Geometry check sheet. Reference: the model listing, model coordinates, mm. A direction names the side the tool comes from. Coordinates: 2 decimals unless noted, no trailing zeros. Loops run counter-clockwise (first coordinate to the right, second up) from the corner with the lowest first, then second, coordinate; pieces in that order, holes last. Notation, with made-up numbers: (60, 59) -> (99, 59) arc R25 ccw to (99, 79) -> close; hole circle Ø9 at (48.5, 49.5). An arc over 180 degrees is marked (long way). Answer as a JSON object with one key per item and string values.
from build123d import *

# Parameters (mm, degrees)
F0_W     = 304.8
F0_H     = 304.8
F1_DEPTH = 152.4
F3_DEPTH = 152.4
F5_DEPTH = 121.92


with BuildPart() as f1:
    # F0 (on Front) → F1 (new body)
    with BuildSketch(Plane.XZ):
        Rectangle(F0_W, F0_H)
    extrude(amount=F1_DEPTH)

    # F2 (on face) → F3 (join)
    with BuildSketch(Plane.XZ.offset(152.4)):
        with BuildLine():
            Line((-152.4, 152.4), (152.4, 152.4))
            ThreePointArc((152.4, 152.4), (0, 304.8), (-152.4, 152.4))
        make_face()
    extrude(amount=-F3_DEPTH)

    # F4 (on face) → F5 (cut)
    with BuildSketch(Plane.XZ.offset(152.4)):
        with BuildLine():
            Line((-121.92, 152.4), (-121.92, -121.92))
            Line((-121.92, -121.92), (121.92, -121.92))
            Line((121.92, -121.92), (121.92, 152.4))
            ThreePointArc((121.92, 152.4), (0, 274.32), (-121.92, 152.4))
        make_face()
    extrude(amount=-F5_DEPTH, mode=Mode.SUBTRACT)


solid = f1.part
1. Section check A-A, the plane y = -35.5. Record the boundary of the cut face in (x, z).
Evaluation:
{"outline": "(-152.4, -152.4) -> (152.4, -152.4) -> (152.4, 152.4) arc R152.4 ccw to (-152.4, 152.4) -> close; hole (-121.92, -121.92) -> (121.92, -121.92) -> (121.92, 152.4) arc R121.92 ccw to (-121.92, 152.4) -> close"}
2. Section check B-B, the plane z = -42. Record the boundary of the cut face in (x, y).
Evaluation:
{"outline": "(-152.4, -152.4) -> (-121.92, -152.4) -> (-121.92, -30.48) -> (121.92, -30.48) -> (121.92, -152.4) -> (152.4, -152.4) -> (152.4, 0) -> (-152.4, 0) -> close"}
3. Section check D-D, the plane y = -10.5. Record the boundary of the cut face in (x, z).
Evaluation:
{"outline": "(-152.4, -152.4) -> (152.4, -152.4) -> (152.4, 152.4) arc R152.4 ccw to (-152.4, 152.4) -> close"}
4. Tool access check on faces 1 (the face through (2.68, -92.29, 274.29)), 2 (the face through (-2, -75, -152.4)). Record the directions out of +Z, -Z, +X, -X, +Y, -Y that give a thin tool (end or side, any length) a straight path to the whole face; none if there is none.
Evaluation:
{"face 1": "-Y", "face 2": "-Z, +X, -X, +Y, -Y"}
5. Mould release check, pull along X, two halves, no side actions. Record for faces 3 (the face through (-2, -92, -121.92)), 4 (the face through (3.351, -77.267, 304.763)), 5 (the face through (-152.4, -75, -2)), 6 (the face through (-125, -152.4, 60)): released by +X, released by -X, zero draft, split by the parting line, or undercut.
Evaluation:
{"face 3": "undercut", "face 4": "split by the parting line", "face 5": "released by -X", "face 6": "zero draft"}
6. Depth check by flat-ended pin: P1, Ø10, axis at y = -125, z = 245, coming from the +X side; P2, Ø1.5, axis at x = -41.5, z = 165, coming from the -Y side; P3, Ø1.5, axis at x = -7.5, y = -105, coming from the +Z side. Enter the tip coordinate at first touch or a pass-through.
Evaluation:
{"P1": "stops at x = 124.71", "P2": "stops at y = -30.48", "P3": "stops at z = 304.65"}
7. Thickness scan on probe 1 along X at (y, z) = (-67.5, 60.5); probe 2 along Y at (x, z) = (-59.5, -57.5); probe 3 along X at (y, z) = (-56.5, 242.5). Record the ranges inside material, lowest first. Write a range as from..to.
Evaluation:
{"probe 1": "x = -152.4..-121.92, 121.92..152.4", "probe 2": "y = -30.48..0", "probe 3": "x = -122.91..-82.14, 82.14..122.91"}
8. Section check C-C, the plane x = 0. Record the boundary of the cut face in (y, z), then the cut area to 3 significant figures.
Evaluation:
{"outline": "(-152.4, -152.4) -> (0, -152.4) -> (0, 304.8) -> (-152.4, 304.8) -> (-152.4, 274.32) -> (-30.48, 274.32) -> (-30.48, -121.92) -> (-152.4, -121.92) -> close", "area": "21,400 mm^2"}
